Input: part model. Units: mm. Frame: model coordinates. A direction names the side the tool comes from. Give positions to 0.01 mm unless a question says otherwise; leave off trailing zeros. Write each loop counter-clockwise with the first axis right and the second up, starting at its lowest first coordinate (ties: lowest second). Pieces come first, ordered by that corner, then holes. Notation, with made-up numbers: (43, 56) -> (101, 56) arc R14 cw to (101, 60) -> close; hole circle Ø3 at (85, -1). An arc over 180 degrees is marked (long way). Return JSON: item names as keys, results as strings. Group by question number.
Item 1: Set-up query: faces 4 (the face through (-29, 3, -1)), 5 (the face through (33, 1, -1)). Return all of +Z, -Z, +X, -X, +Y, -Y with unobstructed straight access to the full face (end or side cutting, diameter ignored); none if empty.
Item 2: Section A-A, the plane x = -16.5. Return loops of the section in (y, z), then the cut area to 3 significant figures.
Item 3: Line query: line 1 (Z direction, x = 14.5, y = 1.75); line 2 (X direction, y = 1.5, z = 34.5); line 3 (Y direction, x = -23, z = -23). Output: solid intervals per line, ascending. Write a range as [from, to].
Item 4: Section C-C, the plane z = -45.5. Return loops of the section in (x, y).
Item 5: Section B-B, the plane y = 4.25. Return loops of the section in (x, z), then the cut area to 3 significant figures.
Item 6: Mould query, pull axis X, two halves, no side actions, for faces 1 (the face through (-33, 1, -1)), 2 (the face through (0, 3, 62)), 3 (the face through (0, 1, -66)). Classes: released by +X, released by -X, zero draft, split by the parting line, or undercut.
Autodesk Inventor part; units mm, degrees
ref_plane "YZ Plane" through (0, 0, 0) normal (1, 0, 0) x (0, 1, 0)
ref_plane "XZ Plane" through (0, 0, 0) normal (0, 1, 0) x (-1, 0, 0)
ref_plane "XY Plane" through (0, 0, 0) normal (0, 0, 1) x (1, 0, 0)
sketch "Sketch1" plane through (0, 0, 0) normal (0, 1, 0) x (-1, 0, 0)
  line L0 (29, 62) -> (-29, 62)
  line L1 (-29, 62) -> (-29, -62)
  line L2 (-29, -62) -> (29, -62)
  line L3 (29, -62) -> (29, 62)
  line L4 (29, 62) -> (33, 62)
  line L5 (33, 62) -> (33, 66)
  line L6 (33, 66) -> (29, 66)
  line L7 (29, 66) -> (29, 62)
  line L8 (29, -62) -> (33, -62)
  line L9 (33, -62) -> (33, -66)
  line L10 (33, -66) -> (29, -66)
  line L11 (29, -66) -> (29, -62)
  line L12 (-29, -62) -> (-29, -66)
  line L13 (-29, -66) -> (-33, -66)
  line L14 (-33, -66) -> (-33, -62)
  line L15 (-33, -62) -> (-29, -62)
  line L16 (-29, 62) -> (-33, 62)
  line L17 (-33, 62) -> (-33, 66)
  line L18 (-33, 66) -> (-29, 66)
  line L19 (-29, 66) -> (-29, 62)
  line L20 (29, 66) -> (-29, 66)
  line L21 (-33, 62) -> (-33, -62)
  line L22 (-29, -66) -> (29, -66)
  line L23 (33, -62) -> (33, 62)
  line L24 (-33, 66) -> (-32.8039, 66)
  point P0 (0, 0)
  dimension "d2" = 58
  dimension "d3" = 124
  dimension "d5" = 4
  dimension "d6" = 4
  dimension "d7" = 4
  dimension "d8" = 4
  dimension "d9" = 4
  dimension "d10" = 4
  dimension "d11" = 4
extrude "Extrusion1" add sketch "Sketch1" against normal blind 4
extrude "Extrusion2" add sketch "Sketch1" along normal blind 6 contours L4 L23 L8 L3 | L7 L6 L5 L4 | L0 L19 L20 L7 | L1 L15 L21 L16 | L16 L17 L18 L19 | L11 L22 L12 L2 | L8 L9 L10 L11 | L12 L13 L14 L15
properties part number "Deksel sensor" material "ABS Plastic"
Answer below:
{
 "1": {"face 4": "+Y", "face 5": "+Z, -Z, +X, +Y, -Y"},
 "2": {"outline": "(-4, -66) -> (6, -66) -> (6, -62) -> (0, -62) -> (0, 62) -> (6, 62) -> (6, 66) -> (-4, 66) -> close", "area": "576 mm2"},
 "3": {"line 1": "z = [-66, -62], [62, 66]", "line 2": "x = [-33, -29], [29, 33]", "line 3": "y = [-4, 0]"},
 "4": {"outline": "(-33, -4) -> (33, -4) -> (33, 6) -> (29, 6) -> (29, 0) -> (-29, 0) -> (-29, 6) -> (-33, 6) -> close"},
 "5": {"outline": "(-33, -66) -> (33, -66) -> (33, 66) -> (-33, 66) -> close; hole (-29, -62) -> (29, -62) -> (29, 62) -> (-29, 62) -> close", "area": "1,520 mm2"},
 "6": {"face 1": "released by -X", "face 2": "undercut", "face 3": "zero draft"}
}
